```python
from build123d import *

# Parameters (mm, degrees)
Y_KSEKLIK_EKSTR_ZYON2_DEPTH = 100
KES_EKSTR_ZYON1_DEPTH       = 51.5


with BuildPart() as part:
    # Model → Y_kseklik-Ekstr_zyon2 (new, symmetric)
    with BuildSketch(Plane.XY):
        with BuildLine():
            ThreePointArc((4.999999999999625, 24.392826814455216), (-2.914e-13, 24.900000000000027), (-5.0000000000002, 24.392826814455084))
            Line((-4.9999999999999725, 24.39282681445504), (-4.9999999999999725, 21.000000000000036))
            ThreePointArc((-4.9999999999999725, 21.000000000000036), (-4.843352342230118, 20.718418144374848), (-4.605290303802033, 20.501270047534074))
            Line((-4.605290303802033, 20.501270047534074), (-0.6052903037980408, 20.501270047534074))
            Line((-0.6052903037980408, 20.501270047534074), (3.9683128811226114, 20.353896764673696))
            ThreePointArc((3.9683128811226114, 20.353896764673696), (4.684485734030437, 20.62386506352521), (4.99999999999997, 21.32117215914135))
            Line((4.99999999999997, 21.32117215914135), (4.99999999999997, 24.39282681445528))
        make_face()
        with BuildLine():
            ThreePointArc((4.60529030380189, -20.501270047534113), (4.843352342229974, -20.71841814437489), (4.999999999999826, -21.000000000000078))
            Line((4.999999999999826, -21.000000000000078), (4.999999999999802, -24.39282681445506))
            ThreePointArc((4.999999999999955, -24.39282681445509), (19.293910956568656, -15.740235068130339), (24.900000000000027, 2.166e-14))
            ThreePointArc((24.900000000000027, 2.776e-14), (19.293910956568553, 15.740235068130524), (4.999999999999625, 24.392826814455216))
            Line((4.99999999999997, 24.39282681445528), (4.99999999999997, 21.32117215914135))
            ThreePointArc((4.99999999999997, 21.32117215914135), (4.684485734030437, 20.62386506352521), (3.9683128811226114, 20.353896764673696))
            Line((3.9683128811226114, 20.353896764673696), (-0.6052903037980408, 20.501270047534074))
            Line((-0.6052903037980408, 20.501270047534074), (-4.605290303802033, 20.501270047534074))
            ThreePointArc((-4.605290303802033, 20.501270047534074), (-4.843352342230118, 20.718418144374848), (-4.9999999999999725, 21.000000000000036))
            Line((-4.9999999999999725, 21.000000000000036), (-4.9999999999999725, 24.39282681445504))
            ThreePointArc((-5.0000000000002, 24.392826814455084), (-24.89999999999997, -3.2305e-13), (-4.999999999999519, -24.39282681445517))
            Line((-5.00000000000014, -24.392826814455283), (-5.000000000000119, -21.321172159141323))
            ThreePointArc((-5.000000000000119, -21.321172159141323), (-4.68448573403058, -20.623865063525184), (-3.9683128811227535, -20.353896764673674))
            Line((-3.968312881122754, -20.353896764673674), (0.6052903037978977, -20.501270047534085))
            Line((0.6052903037978977, -20.501270047534085), (4.60529030380189, -20.501270047534113))
        make_face()
        with BuildLine():
            Line((4.999999999999802, -24.39282681445506), (4.999999999999826, -21.000000000000078))
            ThreePointArc((4.999999999999826, -21.000000000000078), (4.843352342229974, -20.71841814437489), (4.60529030380189, -20.501270047534113))
            Line((4.60529030380189, -20.501270047534113), (0.6052903037978977, -20.501270047534085))
            Line((0.6052903037978977, -20.501270047534085), (-3.968312881122754, -20.353896764673674))
            ThreePointArc((-3.9683128811227535, -20.353896764673674), (-4.68448573403058, -20.623865063525184), (-5.000000000000119, -21.321172159141323))
            Line((-5.000000000000119, -21.321172159141323), (-5.00000000000014, -24.392826814455283))
            ThreePointArc((-4.999999999999519, -24.39282681445517), (2.2222e-13, -24.89999999999997), (4.999999999999955, -24.39282681445509))
        make_face()
    extrude(amount=Y_KSEKLIK_EKSTR_ZYON2_DEPTH, both=True)

    # Model_12 → Kes-Ekstr_zyon1 (cut, symmetric)
    with BuildSketch(Plane.XY):
        with BuildLine():
            ThreePointArc((4.999999999999625, 24.392826814455216), (-2.914e-13, 24.900000000000027), (-5.0000000000002, 24.392826814455084))
            Line((-4.9999999999999725, 24.39282681445504), (-4.9999999999999725, 21.000000000000036))
            ThreePointArc((-4.9999999999999725, 21.000000000000036), (-4.843352342230118, 20.718418144374848), (-4.605290303802033, 20.501270047534074))
            Line((-4.605290303802033, 20.501270047534074), (-0.6052903037980408, 20.501270047534074))
            Line((-0.6052903037980408, 20.501270047534074), (3.9683128811226114, 20.353896764673696))
            ThreePointArc((3.9683128811226114, 20.353896764673696), (4.684485734030437, 20.62386506352521), (4.99999999999997, 21.32117215914135))
            Line((4.99999999999997, 21.32117215914135), (4.99999999999997, 24.39282681445528))
        make_face()
        with BuildLine():
            Line((4.999999999999802, -24.39282681445506), (4.999999999999826, -21.000000000000078))
            ThreePointArc((4.999999999999826, -21.000000000000078), (4.843352342229974, -20.71841814437489), (4.60529030380189, -20.501270047534113))
            Line((4.60529030380189, -20.501270047534113), (0.6052903037978977, -20.501270047534085))
            Line((0.6052903037978977, -20.501270047534085), (-3.968312881122754, -20.353896764673674))
            ThreePointArc((-3.9683128811227535, -20.353896764673674), (-4.68448573403058, -20.623865063525184), (-5.000000000000119, -21.321172159141323))
            Line((-5.000000000000119, -21.321172159141323), (-5.00000000000014, -24.392826814455283))
            ThreePointArc((-4.999999999999519, -24.39282681445517), (2.2222e-13, -24.89999999999997), (4.999999999999955, -24.39282681445509))
        make_face()
    extrude(amount=KES_EKSTR_ZYON1_DEPTH, both=True, mode=Mode.SUBTRACT)


solid = part.part
```
Geometry: final body of the model. Coordinates: model frame, mm. A direction names the side the tool comes from. Coordinates: 2 decimals unless noted, no trailing zeros. Write each loop counter-clockwise with the first axis right and the second up, starting at its lowest first coordinate (ties: lowest second). Pieces come first, ordered by that corner, then holes. Notation, with made-up numbers: M 41.5,78.5 L 77.5,78.5 A18 ccw 77.5,113.5 Z; hole C 11.25,0.25 d4. An arc over 180 degrees is marked long. Use CSV: the item, a comma, the result in double quotes. Start each with the question number.
1. Reachability of faces 1 (the face through (5, -23, 1)), 2 (the face through (-10.87, 22.4, 1.4)), 3 (the face through (0, 23, 51.5)) from +Z, -Z, +X, -X, +Y, -Y: full face, straight path, thin tool, end or side. Return the list, or none.
2. Mould query, pull axis Z, two halves, no side actions, for faces 4 (the face through (3, -20.501, 1)), 5 (the face through (0, 0, -100)), 6 (the face through (0, 0, 100)). Classes: pulls with the +Z half, pulls with the -Z half, needs draft (parallel to the pull), parting line crosses it, or undercut.
3. Cut plane B-B on x = -14. Return the cut outline in (y, z).
4. Cut plane D-D on z = 77. Return the cut outline in (x, y), plus the area to 3 significant figures.
5. Ray query, probe 1 along X at (y, z) = (-1, 4.5); probe 2 along Z at (x, y) = (1.5, 21.5). Return the intervals inside material, ascending.
6. First-contact query: P1, Ø4.5, axis at x = 3.5, z = -20, coming from the -Y side; P2, Ø4.5, axis at x = -2.5, z = -20, coming from the +Y side; P3, Ø8, axis at y = 11.5, z = -47, coming from the +X side. Flat tips, straight axial feed; report the tip coordinate or a pass-through.
7. Cut plane C-C on y = -9.5. Return the cut outline in (x, z).
8. Cut plane A-A on z = 37.5. Return the cut outline in (x, y).
Entries:
1,face 1,"-Y"
1,face 2,"+Z, -Z"
1,face 3,"+Y"
2,face 4,"undercut"
2,face 5,"pulls with the -Z half"
2,face 6,"pulls with the +Z half"
3,outline,"M -20.59,-100 L 20.59,-100 L 20.59,100 L -20.59,100 Z"
4,outline,"C 0,0 d49.8"
4,area,"1,950 mm²"
5,probe 1,"-24.88 to 24.88"
5,probe 2,"-100 to -51.5, 51.5 to 100"
6,P1,"y = -24.39"
6,P2,"y = 20.62"
6,P3,"x = 23.74"
7,outline,"M -23.02,-100 L 23.02,-100 L 23.02,100 L -23.02,100 Z"
8,outline,"M -5,-24.39 L -5,-21.32 A1 cw -3.97,-20.35 L 0.61,-20.5 L 4.61,-20.5 A1 cw 5,-21 L 5,-24.39 A24.9 ccw 5,24.39 L 5,21.32 A1 cw 3.97,20.35 L -0.61,20.5 L -4.61,20.5 A1 cw -5,21 L -5,24.39 A24.9 ccw Z"
